```python
from build123d import *

# Parameters (mm, degrees)
EXTRUDE_1_DEPTH      = 1.5
EXTRUDE_2_DEPTH      = 6
EXTRUDE_2_DEPTH_BACK = 1.5
CUT_EXTRUDE_1_REACH  = 52.165
SKETCH_4_W           = 20
SKETCH_4_H           = 19.175354044
CUT_EXTRUDE_2_DEPTH  = 7
FILLET_1_R           = 1
SKETCH_5_W           = 35.5
SKETCH_5_H           = 24
CUT_EXTRUDE_3_DEPTH  = 7
SKETCH_6_R           = 1.5
CUT_EXTRUDE_4_DEPTH  = 7
CUT_EXTRUDE_5_DEPTH  = 7
CUT_EXTRUDE_6_DEPTH  = 7
SKETCH_9_R           = 1.75
CUT_EXTRUDE_7_DEPTH  = 10


with BuildPart() as part:
    # 草图1 → 凸台-拉伸1 (new body)
    with BuildSketch(Plane(origin=(0, 0, 0), x_dir=(1, 0, 0), z_dir=(0, 1, 0))):
        with BuildLine():
            Line((-13.25, 21.25), (13.25, 21.25))
            ThreePointArc((13.25, 21.25), (16.785533906, 19.785533906), (18.25, 16.25))
            Line((18.25, 16.25), (18.25, -16.25))
            ThreePointArc((18.25, -16.25), (16.785533906, -19.785533906), (13.25, -21.25))
            Line((13.25, -21.25), (-13.25, -21.25))
            ThreePointArc((-13.25, -21.25), (-16.785533906, -19.785533906), (-18.25, -16.25))
            Line((-18.25, -16.25), (-18.25, 16.25))
            ThreePointArc((-18.25, 16.25), (-16.785533906, 19.785533906), (-13.25, 21.25))
        make_face()
    extrude(amount=EXTRUDE_1_DEPTH)

    # 草图2 → 凸台-拉伸2 (add, two sides: drawn at the far end of the back side and taken through both)
    with BuildSketch(Plane(origin=(0, 1.5, 0), x_dir=(1, 0, 0), z_dir=(0, 1, 0)).offset(-EXTRUDE_2_DEPTH_BACK)):
        with BuildLine():
            Line((-13.25, -22.75), (13.25, -22.75))
            ThreePointArc((13.25, -22.75), (17.846194078, -20.846194078), (19.75, -16.25))
            Line((19.75, -16.25), (19.75, 16.25))
            ThreePointArc((19.75, 16.25), (17.846194078, 20.846194078), (13.25, 22.75))
            Line((13.25, 22.75), (-13.25, 22.75))
            ThreePointArc((-13.25, 22.75), (-17.846194078, 20.846194078), (-19.75, 16.25))
            Line((-19.75, 16.25), (-19.75, -16.25))
            ThreePointArc((-19.75, -16.25), (-17.846194078, -20.846194078), (-13.25, -22.75))
        make_face()
        with BuildLine():
            Line((-13.25, -21.25), (13.25, -21.25))
            ThreePointArc((13.25, -21.25), (16.785533906, -19.785533906), (18.25, -16.25))
            Line((18.25, -16.25), (18.25, 16.25))
            ThreePointArc((18.25, 16.25), (16.785533906, 19.785533906), (13.25, 21.25))
            Line((13.25, 21.25), (-13.25, 21.25))
            ThreePointArc((-13.25, 21.25), (-16.785533906, 19.785533906), (-18.25, 16.25))
            Line((-18.25, 16.25), (-18.25, -16.25))
            ThreePointArc((-18.25, -16.25), (-16.785533906, -19.785533906), (-13.25, -21.25))
        make_face(mode=Mode.SUBTRACT)
    extrude(amount=EXTRUDE_2_DEPTH + EXTRUDE_2_DEPTH_BACK)

    # 草图3 → 切除-拉伸1 (cut, up to next)
    with BuildSketch(Plane(origin=(0, 0, -22.75), x_dir=(-1, 0, 0), z_dir=(0, 0, -1)), mode=Mode.PRIVATE) as cut_extrude_1_sk1:
        with BuildLine():
            Line((-10, 9.5), (10, 9.5))
            Line((10, 9.5), (10, 6.5))
            ThreePointArc((10, 6.5), (9.707106781, 5.792893219), (9, 5.5))
            Line((9, 5.5), (-9, 5.5))
            ThreePointArc((-9, 5.5), (-9.707106781, 5.792893219), (-10, 6.5))
            Line((-10, 6.5), (-10, 9.5))
        make_face()
    cut_extrude_1_tool1 = extrude(cut_extrude_1_sk1.sketch, amount=-CUT_EXTRUDE_1_REACH, mode=Mode.PRIVATE) & part.part
    add(cut_extrude_1_tool1.solids().sort_by_distance((0, 7.509583, -22.75))[0], mode=Mode.SUBTRACT)

    # 草图4 → 切除-拉伸2 (cut)
    with BuildSketch(Plane.XY.offset(22.75)):
        with Locations((0, 7.5)):
            Rectangle(SKETCH_4_W, SKETCH_4_H)
    extrude(amount=-CUT_EXTRUDE_2_DEPTH, mode=Mode.SUBTRACT)

    # 圆角1
    fillet_1_edges = [part.edges().sort_by_distance(p)[0] for p in [
        (10, 0.75, 15.75),
        (-10, 0.75, 15.75),
        (-10, 3.75, 22.75),
        (10, 3.75, 22.75),
        (-17.846194078, 0, 20.846194078),
        (-19.75, 0, 0),
        (-17.846194078, 0, -20.846194078),
        (0, 0, -22.75),
        (17.846194078, 0, -20.846194078),
        (19.75, 0, 0),
        (17.846194078, 0, 20.846194078),
        (-11.625, 0, 22.75),
        (11.625, 0, 22.75),
    ]]
    fillet(fillet_1_edges, radius=FILLET_1_R)

    # 草图5 → 切除-拉伸3 (cut)
    with BuildSketch(Plane.XZ):
        Rectangle(SKETCH_5_W, SKETCH_5_H)
    extrude(amount=-CUT_EXTRUDE_3_DEPTH, mode=Mode.SUBTRACT)

    # 草图6 → 切除-拉伸4 (cut)
    with BuildSketch(Plane.XZ):
        with Locations(Location((-15.2, 14.25, 0), (0, 0, 270))):
            Circle(SKETCH_6_R)
        with Locations(Location((-15.2, -14.25, 0), (0, 0, 90))):
            Circle(SKETCH_6_R)
        with Locations(Location((15.2, -14.25, 0), (0, 0, 270))):
            Circle(SKETCH_6_R)
        with Locations(Location((15.2, 14.25, 0), (0, 0, 90))):
            Circle(SKETCH_6_R)
    extrude(amount=-CUT_EXTRUDE_4_DEPTH, mode=Mode.SUBTRACT)

    # 草图7 → 切除-拉伸5 (cut)
    with BuildSketch(Plane.ZY.offset(19.75)):
        with BuildLine():
            Line((-11.5, 10.6), (11.5, 10.6))
            Line((11.5, 10.6), (11.5, 5.4))
            ThreePointArc((11.5, 5.4), (11.207106781, 4.692893219), (10.5, 4.4))
            Line((10.5, 4.4), (-10.5, 4.4))
            ThreePointArc((-10.5, 4.4), (-11.207106781, 4.692893219), (-11.5, 5.4))
            Line((-11.5, 5.4), (-11.5, 10.6))
        make_face()
    extrude(amount=-CUT_EXTRUDE_5_DEPTH, mode=Mode.SUBTRACT)

    # 草图8 → 切除-拉伸6 (cut)
    with BuildSketch(Plane(origin=(19.75, 0, 0), x_dir=(0, 0, -1), z_dir=(1, 0, 0))):
        with BuildLine():
            Line((1.3, 10.6), (12.3, 10.6))
            Line((12.3, 10.6), (12.3, 5.4))
            ThreePointArc((12.3, 5.4), (12.007106781, 4.692893219), (11.3, 4.4))
            Line((11.3, 4.4), (2.3, 4.4))
            ThreePointArc((2.3, 4.4), (1.592893219, 4.692893219), (1.3, 5.4))
            Line((1.3, 5.4), (1.3, 10.6))
        make_face()
        with BuildLine():
            Line((-12.2, 10.6), (-3.2, 10.6))
            Line((-3.2, 10.6), (-3.2, 5.4))
            ThreePointArc((-3.2, 5.4), (-3.492893219, 4.692893219), (-4.2, 4.4))
            Line((-4.2, 4.4), (-11.2, 4.4))
            ThreePointArc((-11.2, 4.4), (-11.907106781, 4.692893219), (-12.2, 5.4))
            Line((-12.2, 5.4), (-12.2, 10.6))
        make_face()
    extrude(amount=-CUT_EXTRUDE_6_DEPTH, mode=Mode.SUBTRACT)

    # 草图9 → 切除-拉伸7 (cut)
    with BuildSketch(Plane.XZ):
        with Locations(Location((12.871040469, -18.289006858, 0), (0, 0, 270))):
            Circle(SKETCH_9_R)
    extrude(amount=-CUT_EXTRUDE_7_DEPTH, mode=Mode.SUBTRACT)


solid = part.part
```
Input: part model. Units: mm. Frame: model coordinates. A direction names the side the tool comes from. Round coordinates to 2 decimals unless told otherwise and drop trailing zeros. Write each loop counter-clockwise with the first axis right and the second up, starting at its lowest first coordinate (ties: lowest second). Pieces come first, ordered by that corner, then holes. Notation, with made-up numbers: (61, 41.5) -> (72, 41.5) arc R19 cw to (72, 48.5) -> close; hole circle Ø5 at (26, 46.25). An arc over 180 degrees is marked (long way). Answer as CSV lines item,"result".
1. Section B-B (x = -4.5). Return the cut outline in (y, z), plus the area to 3 significant figures.
Geometry says:
outline,"(0, -21.75) arc R1 ccw to (1, -22.75) -> (5.5, -22.75) -> (5.5, -21.25) -> (1.5, -21.25) -> (1.5, -12) -> (0, -12) -> close; (0, 12) -> (1.5, 12) -> (1.5, 15.75) -> (0, 15.75) -> close"
area,"27.5 mm^2"
2. Section D-D (y = 7). Give the number of separate pieces and of enclosed holes in the cut face, plus the area to 3 significant figures.
Geometry says:
separate pieces,"5"
enclosed holes,"0"
area,"106 mm^2"
3. Reachability of faces 4 (the cylindrical face through (16.82, 4.46, -19.75)), 5 (the flat face through (19, 6, 3.2)), 6 (the cylindrical face through (10.301, 3.802, 22.465)) from +Z, -Z, +X, -X, +Y, -Y: full face, straight path, thin tool, end or side. Return the list, or none.
Geometry says:
face 4,"+Y"
face 5,"+X, -X, +Y"
face 6,"+Z, +Y, -Y"
4. Section C-C (z = -4). Return the cut outline in (x, y), plus the area to 3 significant figures.
Geometry says:
outline,"(-19.75, 1) arc R1 ccw to (-18.75, 0) -> (-17.75, 0) -> (-17.75, 1.5) -> (-18.25, 1.5) -> (-18.25, 4.4) -> (-19.75, 4.4) -> close; (17.75, 0) -> (18.75, 0) arc R1 ccw to (19.75, 1) -> (19.75, 4.4) -> (18.25, 4.4) -> (18.25, 1.5) -> (17.75, 1.5) -> close"
area,"14.3 mm^2"
5. Contact query for flat-ended pins moving along their axis: P1, Ø1.2, axis at x = -8, y = 0.5, coming from the +Z side; P2, Ø1.1, axis at y = 7, z = -22.5, coming from the -X side; P3, Ø5.5, axis at x = 12.87, z = -18.29, coming from the +Y side. Output: stop coordinate, or through.
Geometry says:
P1,"stops at z = 15.75"
P2,"stops at x = -16.37"
P3,"stops at y = 1.5"
6. Mould query, pull axis X, two halves, no side actions, for faces 1 (the flat face through (10, 1, 20)), 2 (the flat face through (19, 6, -12.3)), 3 (the cylindrical face through (-19.449, 0.285, 0.227)). Classes: +X half, -X half, draft (parallel to the pull), parting line (faces both ways), or undercut.
Geometry says:
face 1,"undercut"
face 2,"draft"
face 3,"-X half"
7. Section A-A (z = -14.25). Return the cut outline in (x, y).
Geometry says:
outline,"(-19.75, 1) arc R1 ccw to (-18.75, 0) -> (-16.7, 0) -> (-16.7, 1.5) -> (-18.25, 1.5) -> (-18.25, 7.5) -> (-19.75, 7.5) -> close; (-13.7, 0) -> (13.7, 0) -> (13.7, 1.5) -> (-13.7, 1.5) -> close; (16.7, 0) -> (18.75, 0) arc R1 ccw to (19.75, 1) -> (19.75, 7.5) -> (18.25, 7.5) -> (18.25, 1.5) -> (16.7, 1.5) -> close"
8. Ray query, L1, parallel to X at y = 0.95, z = 14.25; L2, parallel to Z at x = 13.5, y = 5.25; L3, parallel to X at y = 1, z = 0. Return the intervals inside material, ascending. Write a range as [from, to].
Geometry says:
L1,"x = [-19.75, -16.7], [-13.7, 13.7], [16.7, 19.75]"
L2,"z = [-22.75, -21.24], [21.24, 22.75]"
L3,"x = [-19.75, -17.75], [17.75, 19.75]"
